from build123d import *

# Parameters (mm, degrees)
F0_W     = 100
F0_H     = 100
F1_DEPTH = 100
F2_T     = -2.5
F3_W     = 94.9397633225
F3_H     = 2.5
F4_DEPTH = 50
F5_R     = 50
F6_W     = 5.7191289961
F6_H     = 50.7341860794
F7_DEPTH = 100.001


with BuildPart() as f1:
    # F0 (on Top) → F1 (new body)
    with BuildSketch(Plane.XY):
        with Locations((-8.5391569883, -0.5041474987)):
            Rectangle(F0_W, F0_H)
    extrude(amount=F1_DEPTH)

    # F2
    f2_openings = [f1.faces().sort_by_distance(p)[0] for p in [
        (-8.539157, -0.504147, 100),
    ]]
    offset(amount=F2_T, openings=f2_openings)

    # F3 (on face) → F4 (cut)
    with BuildSketch(Plane.XY.offset(100)):
        with Locations((-8.569275327, -49.2541474987)):
            Rectangle(F3_W, F3_H)
    extrude(amount=-F4_DEPTH, mode=Mode.SUBTRACT)

    # F5
    f5_edges = [f1.edges().sort_by_distance(p)[0] for p in [
        (-57.289157, -50.504147, 100),
        (40.180725, -50.504147, 100),
    ]]
    fillet(f5_edges, radius=F5_R)

    # F6 (on face) → F7 (cut, through all)
    with BuildSketch(Plane.YZ.offset(41.4608430117)):
        with Locations((-33.6690526456, 32.1479656268)):
            Rectangle(F6_W, F6_H)
        with Locations((-19.6690526456, 32.1479656268)):
            Rectangle(F6_W, F6_H)
        with Locations((-5.6690526456, 32.1479656268)):
            Rectangle(F6_W, F6_H)
        with Locations((8.3309473544, 32.1479656268)):
            Rectangle(F6_W, F6_H)
        with Locations((22.3309473544, 32.1479656268)):
            Rectangle(F6_W, F6_H)
        with Locations((36.3309473544, 32.1479656268)):
            Rectangle(F6_W, F6_H)
    extrude(amount=-F7_DEPTH, mode=Mode.SUBTRACT)


solid = f1.part
The model under review builds one solid part; all positions refer to its coordinate system, in mm. A direction names the side the tool comes from. Round coordinates to 2 decimals unless told otherwise and drop trailing zeros. Loops run counter-clockwise (first coordinate to the right, second up) from the corner with the lowest first, then second, coordinate; pieces in that order, holes last. Notation, with made-up numbers: (-8.5, -15) - (25.5, -15) arc R22 ccw to (25.5, -3) - close; hole circle Ø4 at (65.5, -37.75). An arc over 180 degrees is marked (long way). Use CSV: the item, a comma, the result in double quotes.
(1) Machinability: for faces 4 (the flat face through (-56.039, -2, 52)), 5 (the flat face through (-58.539, -1, 49)), which of the approach directions +Z, -Z, +X, -X, +Y, -Y give a long, thin tool a straight path to every point of the face, cutting with its end or side? Answer none if there is none.
Working result:
face 4,"+Z"
face 5,"+Z, -Z, -X, +Y, -Y"
(2) The part is to be moulded in two halves that separate along Y. For faces 1 (the flat face through (-9, 49, 100)), 2 (the cylindrical face through (40.2, -35.47, 85.74)), 3 (the flat face through (-9, -48.004, 27)), say which applies: pulls with the +Y half, pulls with the -Y half, needs draft (parallel to the pull), parting line crosses it, or undercut.
Working result:
face 1,"needs draft"
face 2,"pulls with the -Y half"
face 3,"undercut"
(3) Take a section at B-B, the plane x = -49. Give the boundary of the cut face in (y, z), plus the area to 4 significant figures.
Working result:
outline,"(-50.5, 0) - (49.5, 0) - (49.5, 100) - (47, 100) - (47, 2.5) - (-48, 2.5) - (-48, 50) - (-50.5, 50) - close"
area,"612.5 mm^2"
(4) Take a section at D-D, the plane y = 30. Give the boundary of the cut face in (x, z).
Working result:
outline,"(-58.54, 0) - (41.46, 0) - (41.46, 100) - (38.96, 100) - (38.96, 2.5) - (-56.04, 2.5) - (-56.04, 100) - (-58.54, 100) - close"
(5) For line 1 (X direction, y = 0, z = 90); line 2 (Y direction, x = 9, z = 41); line 3 (Y direction, x = -15.5, z = 95), list the stretches that pass through material, from the lowest coordinate up.
Working result:
line 1,"x = -58.54 to -56.04, 38.96 to 41.46"
line 2,"y = -50.5 to -48, 47 to 49.5"
line 3,"y = 47 to 49.5"
(6) Take a section at A-A, the plane y = -32.5. Give the boundary of the cut face in (x, z).
Working result:
outline,"(-58.54, 0) - (41.46, 0) - (41.46, 6.78) - (38.96, 6.78) - (38.96, 2.5) - (-56.04, 2.5) - (-56.04, 6.78) - (-58.54, 6.78) - close; (-58.54, 57.52) - (-56.04, 57.52) - (-56.04, 88.42) - (-58.54, 88.42) - close; (38.96, 57.52) - (41.46, 57.52) - (41.46, 88.42) - (38.96, 88.42) - close"
(7) Clearance check with flat-ended pins moving along their axes: P1, Ø6, axis at x = -1, z = 72, coming from the -Y side; P2, Ø1.5, axis at x = -10, y = -2, coming from the +Z side; P3, Ø3, axis at x = 40, y = -21, coming from the +Z side. State where each tip first meets the part, or that it passes through.
Working result:
P1,"stops at y = 47"
P2,"stops at z = 2.5"
P3,"stops at z = 96.25"
(8) Take a section at C-C, the plane z = 44. State how many separate pieces and enclosed holes the cut face has, plus the area to 3 significant figures.
Working result:
separate pieces,"12"
enclosed holes,"0"
area,"803 mm^2"
